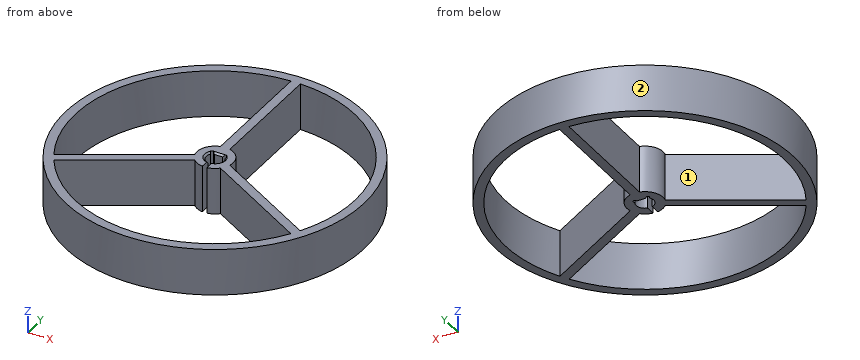
Autodesk Inventor part; units mm, degrees
ref_plane "YZ Plane" through (0, 0, 0) normal (1, 0, 0) x (0, 1, 0)
ref_plane "XZ Plane" through (0, 0, 0) normal (0, 1, 0) x (-1, 0, 0)
ref_plane "XY Plane" through (0, 0, 0) normal (0, 0, 1) x (1, 0, 0)
sketch "スケッチ1" plane through (0, 0, 0) normal (0, 0, 1) x (1, 0, 0)
  circle A0 centre (0, 0) radius 1.5
  circle A1 centre (0, 0) radius 3.1
  line L0 (-0.4, 0) -> (0.4, 0)
  line L1 (0.4, 0) -> (0.4, -3.1)
  line L2 (0.4, -3.1) -> (-0.4, -3.1)
  line L3 (-0.4, -3.1) -> (-0.4, 0)
  line L4 (-1.0712, 1.05) -> (1.0712, 1.05)
  circle A2 centre (0, 0) radius 25.5
  circle A3 centre (0, 0) radius 23.9
  line L5 (-1.4605, 1.0815) -> (-1.1105, 1.4385)
  line L6 (-1.1105, 1.4385) -> (0.175, 0.1785)
  line L7 (0.175, 0.1785) -> (-0.175, -0.1785)
  line L8 (-0.175, -0.1785) -> (-1.4605, 1.0815)
  line L9 (1.4605, 1.0815) -> (1.1105, 1.4385)
  line L10 (1.1105, 1.4385) -> (-0.175, 0.1785)
  line L11 (-0.175, 0.1785) -> (0.175, -0.1785)
  line L12 (0.175, -0.1785) -> (1.4605, 1.0815)
  line L13 (0, 0) -> (-1.0712, 1.05) construction
  line L14 (1.0712, 1.05) -> (0, 0) construction
  point P0 (0.4, -1.4457)
  point P1 (0.4, -3.0741)
  point P2 (-0.4, -3.0741)
  point P3 (-0.4, -1.4457)
  point P4 (-0.7141, 1.05)
  point P5 (0.7141, 1.05)
  point P6 (1.2312, 0.8568)
  point P7 (-1.2312, 0.8568)
  dimension "SHAFT_D" = 3
  dimension "SLIT" = 0.8
  dimension "HUB_THIN" = 1.6
  dimension "d3" = 1.05
  dimension "WHEEL_D" = 51
  dimension "d5" = 1.6
  dimension "d18" = 0.5
  dimension "d19" = 1.8
extrude "ハブ＆リム" add sketch "スケッチ1" along normal blind 8 contours A0 L12 L9 L10 L6 L5 L8 L3 A1 L1 | L10 L4 L6 A0 | A2
sketch "スケッチ2" plane through (0, 0, 0) normal (0, 0, 1) x (1, 0, 0)
  line L0 (-0.8, 2.6) -> (0.8, 2.6)
  line L1 (0.8, 2.6) -> (0.8, 23.9)
  line L2 (0.8, 23.9) -> (-0.8, 23.9)
  line L3 (-0.8, 23.9) -> (-0.8, 2.6)
  circle A0 centre (0, 0) radius 23.9
  point P0 (0, 23.9)
  dimension "d8" = 1.6
  dimension "d9" = 2.6
extrude "スポーク" add sketch "スケッチ2" along normal up to surface (8 mm away) contours L3 A0 L1 L0 | L3 L2 A0 | A0 L2 L1 picked at (0, 9.7)
pattern_circular "円形状パターン1" count 3 over 360 about axis through (0, 0, -10) along (0, 0, 1) of "スポーク"
chamfer "面取り1" distance 0.3 angle 45 3 edges at (-1.4109, -0.5094, 8) (0, 1.05, 8) (1.4109, -0.5094, 8)
equation "\"d5\" = HUB_THIN"
properties part number "D-Shaft_Wheel3"
For this review, take the finished solid that the model builds, in its own axes (mm). Face numbers are marked on the shaded views. Give positions to 0.01 mm unless a question says otherwise; leave off trailing zeros. Write each loop counter-clockwise with the first axis right and the second up, starting at its lowest first coordinate (ties: lowest second). Pieces come first, ordered by that corner, then holes. Notation, with made-up numbers: M 55.5,17 L 103.5,17 A20 ccw 103.5,42 Z; hole C 17.25,-27 d2. An arc over 180 degrees is marked long. One line per item, written item: value.
1) The part is to be moulded in two halves that separate along X. For the marked faces 1 and 2, say which applies: +X half, -X half, draft (parallel to the pull), parting line (faces both ways), or undercut.
Results are:
face 1: undercut
face 2: parting line
2) Take a section at C-C, the plane z = 5.25. Count the separate pieces of the cut face and the enclosed holes in it, then the cut area to 3 significant figures.
Results are:
separate pieces: 1
enclosed holes: 3
area: 370 mm²
3) Take a section at A-A, the plane y = 0. Write out the cut boundary in (x, z), then the cut area to 3 significant figures.
Results are:
outline: M -25.5,0 L -23.9,0 L -23.9,8 L -25.5,8 Z; M -3.1,0 L -1.5,0 L -1.5,7.7 L -1.8,8 L -3.1,8 Z; M 1.5,0 L 3.1,0 L 3.1,8 L 1.8,8 L 1.5,7.7 Z; M 23.9,0 L 25.5,0 L 25.5,8 L 23.9,8 Z
area: 51.1 mm²
4) For line 1 (Y direction, x = -18, z = 4.75); line 2 (Y direction, x = 2.5, z = 2); line 3 (X direction, y = 16.5, z = 0.5), list the stretches that pass through material, from the lowest coordinate up. Write a range as from..to.
Results are:
line 1: y = -18.06..-15.72, -11.32..-9.47, 15.72..18.06
line 2: y = -25.38..-23.77, -2.37..1.83, 23.77..25.38
line 3: x = -19.44..-17.29, -0.8..0.8, 17.29..19.44
5) For P1, Ø1.8, axis at y = -2.5, z = 4, coming from the +X side; P2, Ø3, axis at x = -17.5, z = 4.5, coming from the -Y side; P3, Ø2, axis at x = 10, z = 2.5, coming from the -Y side, all flat-tipped, find the tip position at first contact; note any pin that passes through.
Results are:
P1: stops at x = 25.45
P2: stops at y = -19.86
P3: stops at y = -23.86
6) Take a section at D-D, the plane y = 22. Write out the cut boundary in (x, z).
Results are:
outline: M -12.89,0 L -9.34,0 L -9.34,8 L -12.89,8 Z; M -0.8,0 L 0.8,0 L 0.8,8 L -0.8,8 Z; M 9.34,0 L 12.89,0 L 12.89,8 L 9.34,8 Z
7) Take a section at B-B, the plane x = 13.5. Write out the cut boundary in (y, z), then the cut area to 3 significant figures.
Results are:
outline: M -21.63,0 L -19.72,0 L -19.72,8 L -21.63,8 Z; M -8.72,0 L -6.87,0 L -6.87,8 L -8.72,8 Z; M 19.72,0 L 21.63,0 L 21.63,8 L 19.72,8 Z
area: 45.4 mm²
